Autodesk Inventor part; units mm, degrees
ref_plane "YZ Plane" through (0, 0, 0) normal (1, 0, 0) x (0, 1, 0)
ref_plane "XZ Plane" through (0, 0, 0) normal (0, 1, 0) x (-1, 0, 0)
ref_plane "XY Plane" through (0, 0, 0) normal (0, 0, 1) x (1, 0, 0)
sketch "Sketch1" plane through (0, 0, 0) normal (0, 0, 1) x (1, 0, 0)
  line L0 (0, 0) -> (53.34, 0)
  line L1 (53.34, 0) -> (53.34, 38.1)
  line L2 (53.34, 38.1) -> (0, 38.1)
  line L3 (0, 38.1) -> (0, 0)
  dimension "d0" = 53.34
  dimension "d1" = 38.1
extrude "Extrusion1" add sketch "Sketch1" along normal blind 1.6
sketch "Sketch2" plane through (0, 0, 1.6) normal (0, 0, 1) x (1, 0, 0)
  line L0 (53.34, 38.1) -> (0, 38.1)
  line L1 (0, 0) -> (53.34, 0)
  line L2 (0, 38.1) -> (0, 0)
  line L3 (53.34, 0) -> (53.34, 38.1)
  point P0 (4.318, 33.782)
  point P1 (49.022, 33.782)
  point P2 (49.022, 4.318)
  point P3 (4.318, 4.318)
  dimension "d4" = 29.464
  dimension "d5" = 4.318
  dimension "d6" = 38.1
  dimension "d7" = 53.34
  dimension "d8" = 4.318
  dimension "d9" = 4.318
hole "Hole1" at (4.318, 33.782, 1.6) at (49.022, 33.782, 1.6) at (49.022, 4.318, 1.6) at (4.318, 4.318, 1.6) direction (0, 0, -1) diameter 4.572 end through all
sketch "Sketch3" plane through (0, 0, 1.6) normal (0, 0, 1) x (1, 0, 0)
  line L0 (0, 38.1) -> (0, 0)
  line L1 (53.34, 38.1) -> (0, 38.1)
  line L2 (0, 0) -> (53.34, 0)
  line L3 (53.34, 0) -> (53.34, 38.1)
  point P0 (19.256, 28.194)
  point P1 (31.48, 28.194)
  point P2 (40.878, 28.194)
  point P3 (9.921, 20.526)
  point P4 (43.419, 15.542)
  point P5 (17.574, 10.175)
  point P6 (33.29, 10.175)
  point P7 (17.256, 28.194)
  point P8 (15.256, 28.194)
  point P9 (13.256, 28.194)
  point P10 (38.878, 28.194)
  point P11 (29.48, 28.194)
  point P12 (9.921, 18.526)
  point P13 (9.921, 16.526)
  point P14 (9.921, 14.526)
  point P15 (19.574, 10.175)
  point P16 (21.574, 10.175)
  point P17 (23.574, 10.175)
  point P18 (35.29, 10.175)
  point P19 (43.419, 17.542)
  point P20 (43.419, 19.542)
  point P21 (43.419, 21.542)
  dimension "d17" = 19.256
  dimension "d18" = 31.48
  dimension "d19" = 40.878
  dimension "d20" = 9.906
  dimension "d44" = 2
  dimension "d51" = 2
  dimension "d58" = 2
  dimension "d63" = 9.921
  dimension "d64" = 17.574
  dimension "d65" = 17.574
  dimension "d66" = 10.175
  dimension "d67" = 33.29
  dimension "d68" = 15.542
  dimension "d69" = 9.921
  dimension "d72" = 2
  dimension "d79" = 2
  dimension "d86" = 2
  dimension "d93" = 2
hole "Hole2" at (19.256, 28.194, 1.6) at (31.48, 28.194, 1.6) at (40.878, 28.194, 1.6) at (9.921, 20.526, 1.6) at (43.419, 15.542, 1.6) at (17.574, 10.175, 1.6) at (33.29, 10.175, 1.6) at (17.256, 28.194, 1.6) at (15.256, 28.194, 1.6) at (13.256, 28.194, 1.6) at (38.878, 28.194, 1.6) at (29.48, 28.194, 1.6) at (9.921, 18.526, 1.6) at (9.921, 16.526, 1.6) at (9.921, 14.526, 1.6) at (19.574, 10.175, 1.6) at (21.574, 10.175, 1.6) at (23.574, 10.175, 1.6) at (35.29, 10.175, 1.6) at (43.419, 17.542, 1.6) at (43.419, 19.542, 1.6) at (43.419, 21.542, 1.6) direction (0, 0, -1) diameter 0.8 end through all
sketch "Sketch4" plane through (0, 0, 1.6) normal (0, 0, 1) x (1, 0, 0)
  line L0 (53.34, 38.1) -> (0, 38.1)
  line L1 (0, 38.1) -> (0, 0)
  point P0 (18.557, 17.521)
  point P1 (21.097, 17.521)
  point P2 (23.637, 17.521)
  point P3 (18.557, 20.061)
  point P4 (21.097, 20.061)
  point P5 (23.637, 20.061)
  dimension "d105" = 20.579
  dimension "d106" = 18.557
  dimension "d109" = 2.54
  dimension "d112" = 2.54
hole "Hole3" at (18.557, 17.521, 1.6) at (21.097, 17.521, 1.6) at (23.637, 17.521, 1.6) at (18.557, 20.061, 1.6) at (21.097, 20.061, 1.6) at (23.637, 20.061, 1.6) direction (0, 0, -1) diameter 1 end through all
properties part number "board"
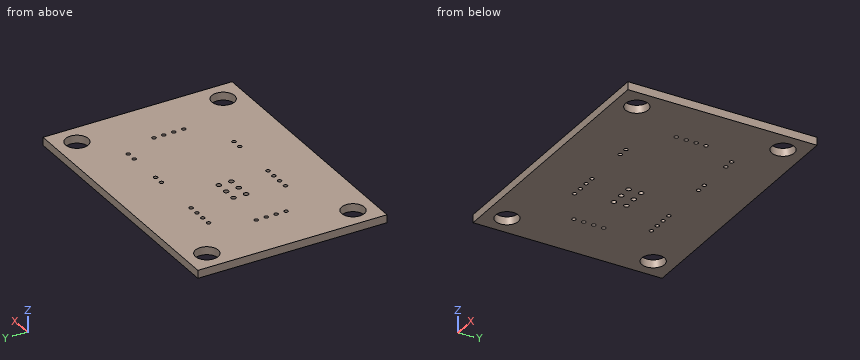
For this review, take the finished solid that the model builds, in its own axes (mm). Coordinates: 2 decimals unless noted, no trailing zeros. Order: outer loops, then holes, each group sorted by start corner. A loop starts at its lowest first (then second) coordinate and runs counter-clockwise, first axis right, second up. Notation, with made-up numbers: (12.5, 5) -> (41.5, 5) arc R13 cw to (41.5, 14) -> close; hole circle Ø9 at (74.5, 17). An arc over 180 degrees is marked (long way). Answer as CSV lines item,"result".
Q1. Clearance check with a flat-ended pin moving along its axis: pin 1 Ø2.5 at (x, y) = (49.022, 4.318) entering from -Z. State where the tip first meets the part, or that it passes through.
Model answer:
pin 1,"passes through"
Q2. Wall thickness on line 1 along X through (y, z) = (5, 0.6); line 2 along Y through (x, z) = (3, 0.35); line 3 along X through (y, z) = (4.5, 0.2): over which ranges is each line inside the solid? List them lowest first. Write a range as [from, to].
Model answer:
line 1,"x = [0, 2.14], [6.5, 46.84], [51.2, 53.34]"
line 2,"y = [0, 2.45], [6.19, 31.91], [35.65, 38.1]"
line 3,"x = [0, 2.04], [6.6, 46.74], [51.3, 53.34]"
Q3. We need section B-B (z = 0.8). Count the separate pieces of the cut face and the enclosed holes in it, plus the area to 3 significant figures.
Model answer:
separate pieces,"1"
enclosed holes,"32"
area,"1,950 mm2"
Q4. We need section A-A (y = 5). State the section outline as (x, z) points.
Model answer:
outline,"(0, 0) -> (2.14, 0) -> (2.14, 1.6) -> (0, 1.6) -> close; (6.5, 0) -> (46.84, 0) -> (46.84, 1.6) -> (6.5, 1.6) -> close; (51.2, 0) -> (53.34, 0) -> (53.34, 1.6) -> (51.2, 1.6) -> close"
